The figure shows three views and two pictorial views of one solid part (mm, origin at its lowest corner). Answer the questions. A direction names the side the tool comes from. Give positions to 0.01 mm unless a question says otherwise; leave off trailing zeros. Loops run counter-clockwise (first coordinate to the right, second up) from the corner with the lowest first, then second, coordinate; pieces in that order, holes last. Notation, with made-up numbers: M 64.25,-28 L 111.25,-28 A38 cw 111.25,10 Z; hole C 68.5,38 d9. An arc over 180 degrees is marked long. One line per item, written item: value. Start each with the question number.
Q1. A cutting plane is placed at B-B, the plane z = 30.5. Determine the outline of the cut face in (x, y).
Q2. For the marked faces 4, 5 and 6, determine the directions among +Z, -Z, +X, -X, +Y, -Y from which every point of the face is accessible in a straight line to the end or side of a thin tool.
Q3. A cutting plane is placed at D-D, the plane z = 11.5. Determine the outline of the cut face in (x, y) (1 decimal), and give its area (3 significant figures).
Q4. Flat-ended cylindrical pins translate along their axes: pin 1 (3 mm diameter, centred on y = 7, z = 5.5, fed in from +X); pin 2 (4 mm diameter, centred on x = 82.5, y = 18, fed in from +Z); pin 3 (3.5 mm diameter, centred on x = 5, z = 40.5, fed in from -Y). Find the tip coordinate at first contact, or state that the pin passes through.
Q5. The mould has two halves that part along X. Classify the marked faces 1, 2 and 3: +X half, -X half, draft (parallel to the pull), parting line (faces both ways), or undercut.
Q6. Consider L1, parallel to X at y = 26.5, z = 26.5; L2, parallel to Z at x = 51, y = 16.5; L3, parallel to Y at x = 72, z = 12 (1 decimal). Determine where each line is inside the solid, lowest interval first.
Q7. A cutting plane is placed at A-A, the plane y = 12.5. State how many separate pieces and enclosed holes the cut face has, and give its area (3 significant figures).
Q8. A cutting plane is placed at C-C, the plane x = 96.5. Determine the outline of the cut face in (y, z) (1 decimal).
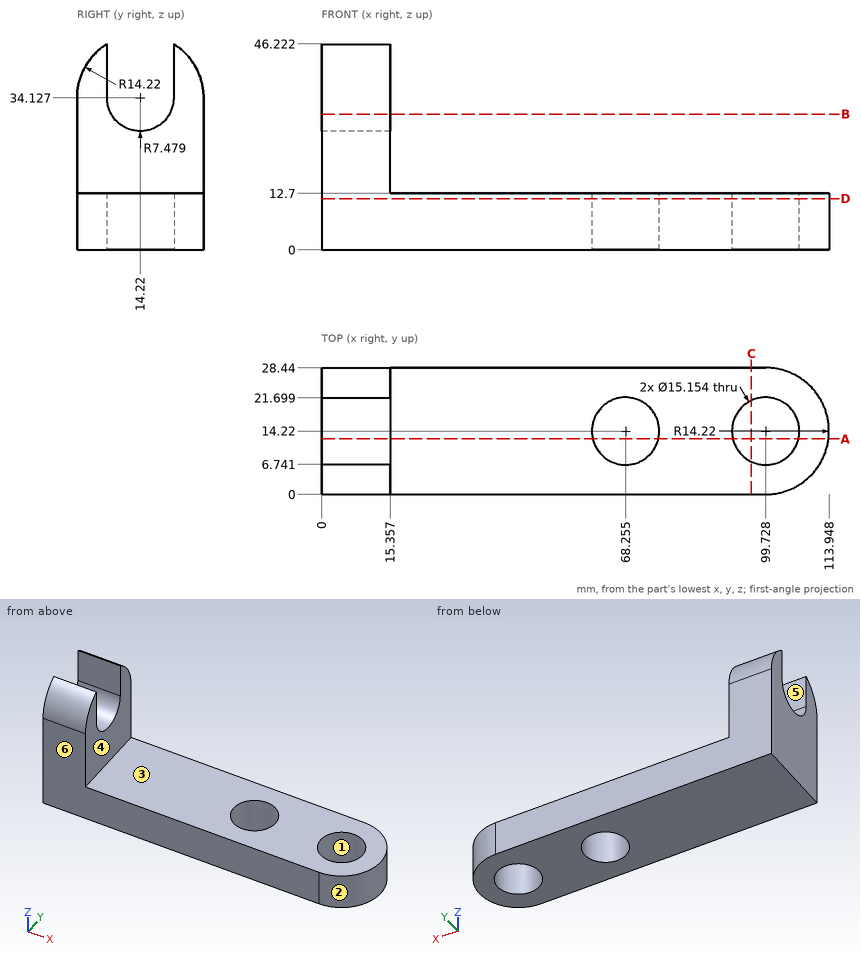
Answer block:
1. outline: M 0,0 L 15.36,0 L 15.36,7.68 L 0,7.68 Z; M 0,20.76 L 15.36,20.76 L 15.36,28.44 L 0,28.44 Z
2. face 4: +Z, +X, +Y, -Y
2. face 5: +Z, +X, -X
2. face 6: +Z, -Z, +X, -X, -Y
3. outline: M 0,0 L 99.7,0 A14.2 ccw 99.7,28.4 L 0,28.4 Z; hole C 68.3,14.2 d15.2; hole C 99.7,14.2 d15.2
3. area: 2,790 mm^2
4. pin 1: x = 112.75
4. pin 2: z = 12.7
4. pin 3: y = 0.77
5. face 1: undercut
5. face 2: +X half
5. face 3: draft
6. L1: 0 to 15.36
6. L2: 0 to 12.7
6. L3: 0 to 7.6, 20.8 to 28.4
7. separate pieces: 3
7. enclosed holes: 0
7. area: 1,290 mm^2
8. outline: M 0,0 L 7.4,0 L 7.4,12.7 L 0,12.7 Z; M 21.1,0 L 28.4,0 L 28.4,12.7 L 21.1,12.7 Z
